Autodesk Inventor part; units mm, degrees
ref_plane "YZ Plane" through (0, 0, 0) normal (1, 0, 0) x (0, 1, 0)
ref_plane "XZ Plane" through (0, 0, 0) normal (0, 1, 0) x (-1, 0, 0)
ref_plane "XY Plane" through (0, 0, 0) normal (0, 0, 1) x (1, 0, 0)
sketch "Sketch1" plane through (0, 0, 0) normal (0, 0, 1) x (1, 0, 0)
  line L0 (0, 0) -> (0, 7) construction
  line L1 (0, 7) -> (10, 7)
  line L2 (0, 7) -> (1.5, 5.5)
  line L3 (10, 7) -> (10, 9)
  line L4 (10, 9) -> (15, 9)
  line L5 (15, 9) -> (15, 5.5)
  line L6 (15, 5.5) -> (1.5, 5.5)
  line L7 (0, 0) -> (19.3515, 0)
  line L8 (2, 4) -> (15, 4)
  line L9 (15, 4) -> (15, 5.5)
  line L10 (1.5, 5.5) -> (1.5, 0) construction
  line L11 (2, 5) -> (2, 4)
  line L12 (2, 5) -> (1.5, 5.5)
  dimension "d0" = 10
  dimension "d1" = 5
  dimension "d2" = 14
  dimension "d3" = 11
  dimension "d4" = 18
  dimension "d8" = 13
  dimension "d9" = 8
  dimension "d10" = 0.5
revolve "Revolution1" add sketch "Sketch1" angle 360 about axis through (0, 0, 0) along (1, 0, 0)
sketch "Sketch2" plane through (15, 0, 0) normal (1, 0, 0) x (0, 0, -1)
  line L0 (-1.5, 9.5651) -> (1.5, 9.5651)
  line L1 (1.5, 9.5651) -> (1.5, 7.5)
  line L2 (1.5, 7.5) -> (-1.5, 7.5)
  line L3 (-1.5, 7.5) -> (-1.5, 9.5651)
  line L4 (8.9736, 1.4966) -> (8.9736, -0.0034)
  line L5 (7.5, -0.0034) -> (7.5, 1.4966)
  line L6 (-1.5, -7.5) -> (1.5, -7.5)
  line L7 (1.5, -7.5) -> (1.5, -9.612)
  line L8 (1.5, -9.612) -> (-1.5, -9.612)
  line L9 (-1.5, -9.612) -> (-1.5, -7.5)
  circle A0 centre (0, 0) radius 7
  circle A1 centre (0, 0) radius 9
  circle A2 centre (0, 0) radius 4
  line L10 (7.2867, -0.0034) -> (9.9612, -0.0034) construction
  line L11 (7.5, 1.4966) -> (9, 1.4966)
  line L12 (7.5, -1.5034) -> (9, -1.5034)
  line L13 (7.5, -0.0034) -> (7.5, -1.5034)
  line L14 (9, 0) -> (9, -1.5034)
  line L15 (-10.5, 1.5) -> (-7.5, 1.5)
  line L16 (-7.5, 1.5) -> (-7.5, -1.5)
  line L17 (-7.5, -1.5) -> (-10.5, -1.5)
  line L18 (-10.5, -1.5) -> (-10.5, 1.5)
  line L19 (-10.5, 1.5) -> (-7.5, -1.5) construction
  line L20 (-7.5, 1.5) -> (-10.5, -1.5) construction
  point P0 (0, 9)
  point P1 (0, -9)
  point P2 (-9, 0)
  point P3 (-1.5, -8.8741)
  point P4 (1.5, -8.8741)
  point P5 (-8.8741, 1.5)
  point P6 (-8.8741, -1.5)
  point P7 (1.5, 8.8741)
  point P8 (-1.5, 8.8741)
  point P9 (8.8736, -1.5034)
  point P10 (8.8747, 1.4966)
  dimension "d11" = 1.5
  dimension "d12" = 1.5
  dimension "d13" = 1.5
  dimension "d16" = 1.5
  dimension "d18" = 1.5
  dimension "d20" = 3
  dimension "d21" = 3
  dimension "d22" = 3
  dimension "d23" = 1.5
  dimension "d24" = 3
  dimension "d25" = 1.5
extrude "Extrusion1" cut sketch "Sketch2" against normal blind 10 contours A1 L1 L2 L3 | L15 L16 L17 A1 | A1 L12 L13 L5 L11 | L9 L6 L7 A1
thread "Thread1"
properties material "Aluminum 6061-AHC"
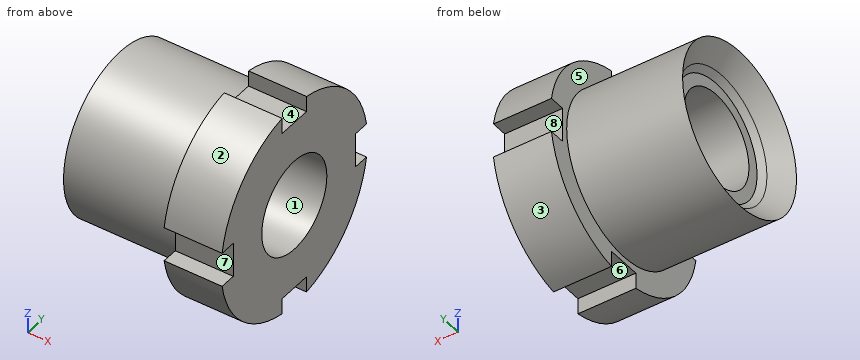
Part model, mm, in its own coordinate system. Face numbers are marked on the shaded views. A direction names the side the tool comes from. Coordinates: 2 decimals unless noted, no trailing zeros. Loops run counter-clockwise (first coordinate to the right, second up) from the corner with the lowest first, then second, coordinate; pieces in that order, holes last. Notation, with made-up numbers: (-26.5, -28.5) - (-4.5, -28.5) arc R19 cw to (-4.5, -23.5) - close; hole circle Ø11 at (-23.75, 30.25). An arc over 180 degrees is marked (long way). Write each question's results on one line, items separated by ' | '. Start each with the question number.
Q1. Which spindle directions (+Z, -Z, +X, -X, +Y, -Y) get a long thin tool onto all of the face, cutting with end or side? Do the marked faces 5, 6, 7 and 8. Say none if no direction does.
Q2. Two-plate mould, pull along Y, no slides. Class the marked faces 1, 2, 3 and 4: +Y half, -Y half, draft (parallel to the pull), parting line (faces both ways), or undercut.
Q3. Slice it at C-C on y = -7.25. Give the cut face in (x, z), and give its area (3 significant figures).
Q4. Probe line 1 along Z through (x, y) = (12, 0); line 2 along Z through (x, y) = (7.25, 0); line 3 along X through (y, z) = (-1, 4). List the from-to ranges inside material, lowest first.
Q5. Slice it at A-A on x = 12.5. Give the cut face in (y, z).
Q6. Drop flat-ended pins along their axis: pin 1 Ø1.5 at (x, y) = (13.5, -8) entering from -Z; pin 2 Ø2 at (x, y) = (6, 3) entering from -Z; pin 3 Ø3 at (x, y) = (8, -5) entering from +Z. Give the stop position or say it passes through.
Q7. Slice it at B-B on x = 6.75. Give the cut face in (y, z), and give its area (3 significant figures).
Answer:
1) face 5: -X | face 6: -Z, +X, -X | face 7: +X, -X, -Y | face 8: +X, -X, +Y
2) face 1: undercut | face 2: -Y half | face 3: +Y half | face 4: undercut
3) outline: (10, -5.33) - (15, -5.33) - (15, 5.33) - (10, 5.33) - close | area: 53.3 mm2
4) line 1: z = -7.5 to -4, 4 to 7.5 | line 2: z = -7 to -4, 4 to 7 | line 3: x = 2 to 15
5) outline: (-8.87, -1.5) arc R9 ccw to (-1.5, -8.87) - (-1.5, -7.5) - (1.5, -7.5) - (1.5, -8.87) arc R9 ccw to (8.87, -1.5) - (7.5, -1.5) - (7.5, 1.5) - (8.87, 1.5) arc R9 ccw to (1.5, 8.87) - (1.5, 7.5) - (-1.5, 7.5) - (-1.5, 8.87) arc R9 ccw to (-8.87, 1.5) - (-7.5, 1.5) - (-7.5, -1.5) - close; hole circle Ø8 at (0, 0)
6) pin 1: stops at z = -5.33 | pin 2: stops at z = -6.71 | pin 3: stops at z = 6.06
7) outline: circle Ø14 at (0, 0); hole circle Ø8 at (0, 0) | area: 104 mm2
